Autodesk Inventor part; units mm, degrees
ref_plane "YZ Plane" through (0, 0, 0) normal (1, 0, 0) x (0, 1, 0)
ref_plane "XZ Plane" through (0, 0, 0) normal (0, 1, 0) x (-1, 0, 0)
ref_plane "XY Plane" through (0, 0, 0) normal (0, 0, 1) x (1, 0, 0)
sketch "Sketch1" plane through (0, 0, 0) normal (0, 0, 1) x (1, 0, 0)
  line L0 (-35, 12.5) -> (35, 12.5)
  line L1 (35, 12.5) -> (35, -12.5)
  line L2 (35, -12.5) -> (-35, -12.5)
  line L3 (-35, -12.5) -> (-35, 12.5)
  point P0 (0, 0)
  dimension "d0" = 70
  dimension "d1" = 25
  dimension "d2" = 35
  dimension "d3" = 12.5
extrude "Extrusion1" add sketch "Sketch1" along normal blind 42
full round fillet "Full Round Fillet1" first side at (11.6667, 12.5, 14) centre faces at (-35, 4.1667, 14) second side at (-11.6667, -12.5, 14)
full round fillet "Full Round Fillet2" first side at (15.8333, 12.5, 14) centre faces at (35, -4.1667, 14) second side at (-3.3334, -12.5, 28)
sketch "Sketch2" plane through (0, 0, 42) normal (0, 0, 1) x (1, 0, 0)
  circle A0 centre (-20, 0) radius 6
  circle A1 centre (20, 0) radius 6
  point P0 (0, 0)
  dimension "d6" = 12
  dimension "d7" = 12
  dimension "d8" = 40
  dimension "d9" = 20
extrude "Extrusion2" cut sketch "Sketch2" against normal blind 42
thread "Thread1"
thread "Thread2"
properties part number "Topo Macaco" material "Steel ASTM A36"
Can you work these out from the model? Positions are in its coordinate system, mm. Give positions to 0.01 mm unless a question says otherwise; leave off trailing zeros. Write each loop counter-clockwise with the first axis right and the second up, starting at its lowest first coordinate (ties: lowest second). Pieces come first, ordered by that corner, then holes. Notation, with made-up numbers: (32, -4.75) -> (89, -4.75) arc R19 cw to (89, 0.25) -> close; hole circle Ø4 at (19, -5.75). An arc over 180 degrees is marked (long way). Answer as a JSON object with one key per item and string values. Group by question number.
Item 1: Please list where these lines run through material, in increasing order: line 1 (Y direction, x = 20, z = 31); line 2 (X direction, y = 5.5, z = 39.5) (3 decimals); line 3 (X direction, y = -2.75, z = 15). Write a range as [from, to].
Item 2: Suppose I cut it at D-D (y = -5). Please give me the cut outline in (x, z).
Item 3: Suppose I cut it at A-A (x = 20). Please give me the cut outline in (y, z), plus the area to 3 significant figures.
Item 4: I'm going to push flat-ended pins straight in: P1, Ø2, axis at y = -1.5, z = 19, coming from the +X side; P2, Ø1.5, axis at x = 27.5, z = 12.5, coming from the -Y side. Where does each tip first touch, or does it pass through?
Item 5: We'd pull the mould along X, two halves only. Please class faces 1 (the face through (-31.436, -8.741, 21.294)), 2 (the face through (31.436, 8.741, 21.294)), 3 (the face through (25.54, -2.3, 21.29)), 4 (the face through (0, -12.5, 21)): +X half, -X half, draft (parallel to the pull), parting line (faces both ways), or undercut.
Item 6: Suppose I cut it at B-B (z = 39.5). State how many separate pieces and enclosed holes the cut face has, plus the area to 3 significant figures.
Item 7: Suppose I cut it at C-C (y = 3). Please give me the cut outline in (x, z).
Findings:
{
 "1": {"line 1": "y = [-12.5, -6], [6, 12.5]", "line 2": "x = [-33.725, -22.398], [-17.602, 17.602], [22.398, 33.725]", "line 3": "x = [-34.69, -25.33], [-14.67, 14.67], [25.33, 34.69]"},
 "2": {"outline": "(-33.96, 0) -> (-23.32, 0) -> (-23.32, 42) -> (-33.96, 42) -> close; (-16.68, 0) -> (16.68, 0) -> (16.68, 42) -> (-16.68, 42) -> close; (23.32, 0) -> (33.96, 0) -> (33.96, 42) -> (23.32, 42) -> close"},
 "3": {"outline": "(-12.5, 0) -> (-6, 0) -> (-6, 42) -> (-12.5, 42) -> close; (6, 0) -> (12.5, 0) -> (12.5, 42) -> (6, 42) -> close", "area": "546 mm²"},
 "4": {"P1": "stops at x = 34.99", "P2": "stops at y = -11.76"},
 "5": {"face 1": "-X half", "face 2": "+X half", "face 3": "undercut", "face 4": "draft"},
 "6": {"separate pieces": "1", "enclosed holes": "2", "area": "1,390 mm²"},
 "7": {"outline": "(-34.63, 0) -> (-25.2, 0) -> (-25.2, 42) -> (-34.63, 42) -> close; (-14.8, 0) -> (14.8, 0) -> (14.8, 42) -> (-14.8, 42) -> close; (25.2, 0) -> (34.63, 0) -> (34.63, 42) -> (25.2, 42) -> close"}
}
